Here's how the part is built. I have some questions about the finished solid (model axes, mm). Face numbers are marked on the shaded views. A direction names the side the tool comes from. Round coordinates to 2 decimals unless told otherwise and drop trailing zeros. Order: outer loops, then holes, each group sorted by start corner. A loop starts at its lowest first (then second) coordinate and runs counter-clockwise, first axis right, second up. Notation, with made-up numbers: (-5, -5.5) -> (39, -5.5) arc R18 cw to (39, 2.5) -> close; hole circle Ø6 at (-22.75, 39). An arc over 180 degrees is marked (long way). One line per item, written item: value.
```python
from build123d import *

# Parameters (mm, degrees)
SKETCH1_W           = 248.68
SKETCH1_H           = 10
BOSS_EXTRUDE1_DEPTH = 80
SKETCH3_W           = 10
SKETCH3_H           = 248.68
BOSS_EXTRUDE2_DEPTH = 40
SKETCH5_W           = 10
SKETCH5_H           = 248.68
BOSS_EXTRUDE3_DEPTH = 50
FILLET1_R           = 11
FILLET2_R           = 11
SKETCH6_W           = 227.416539417
SKETCH6_H           = 3
CUT_EXTRUDE2_DEPTH  = 70


with BuildPart() as part:
    # Sketch1 → Boss-Extrude1 (new body)
    with BuildSketch(Plane(origin=(0, 0, 0), x_dir=(0, 0, -1), z_dir=(1, 0, 0))):
        with Locations((117.31979798, -0.946969697)):
            Rectangle(SKETCH1_W, SKETCH1_H)
    extrude(amount=BOSS_EXTRUDE1_DEPTH)

    # Sketch3 → Boss-Extrude2 (add)
    with BuildSketch(Plane(origin=(0, 4.053030303, 0), x_dir=(1, 0, 0), z_dir=(0, 1, 0))):
        with Locations((5, 117.31979798)):
            Rectangle(SKETCH3_W, SKETCH3_H)
    extrude(amount=BOSS_EXTRUDE2_DEPTH)

    # Sketch5 → Boss-Extrude3 (add)
    with BuildSketch(Plane.XZ.offset(5.946969697)):
        with Locations((5, -117.31979798)):
            Rectangle(SKETCH5_W, SKETCH5_H)
    extrude(amount=BOSS_EXTRUDE3_DEPTH)

    # Fillet1
    # the kernel refuses this fillet: 11 mm, written as the material it takes off along each edge
    with BuildSketch(Plane(origin=(10, 44.053030303, -269.045925855), x_dir=(-1, 0, 0), z_dir=(0, 0, 1))) as fillet1_piece_1:
        with BuildLine():
            CenterArc((11, 10.95445115), FILLET1_R, 180, 84.78409143)
            Line((0, 10.95445115), (-0.22, 10.95445115))
            Line((-0.22, 10.95445115), (-0.22, 0))
            Line((-0.22, 0), (0, -0.22))
            ThreePointArc((0, -0.22), (5, -0.22), (9.98, -0.219089023))
            Line((9.98, -0.219089023), (10, 0))
        make_face()
    extrude(amount=303.452255751, mode=Mode.SUBTRACT)

    # Fillet2
    # the kernel refuses this fillet: 11 mm, written as the material it takes off along each edge
    with BuildSketch(Plane(origin=(10, -55.946969697, 34.406329895), x_dir=(-1, 0, 0), z_dir=(0, 0, -1))) as fillet2_piece_1:
        with BuildLine():
            CenterArc((11, 10.95445115), FILLET2_R, 180, 84.78409143)
            Line((0, 10.95445115), (-0.22, 10.95445115))
            Line((-0.22, 10.95445115), (-0.22, 0))
            Line((-0.22, 0), (0, -0.22))
            ThreePointArc((0, -0.22), (5, -0.22), (9.98, -0.219089023))
            Line((9.98, -0.219089023), (10, 0))
        make_face()
    extrude(amount=303.452255751, mode=Mode.SUBTRACT)

    # Sketch6 → Cut-Extrude2 (cut)
    with BuildSketch(Plane(origin=(80, 0, 0), x_dir=(0, 0, -1), z_dir=(1, 0, 0))):
        with Locations((117.951528272, -0.946969697)):
            Rectangle(SKETCH6_W, SKETCH6_H)
    extrude(amount=-CUT_EXTRUDE2_DEPTH, mode=Mode.SUBTRACT)


solid = part.part
```
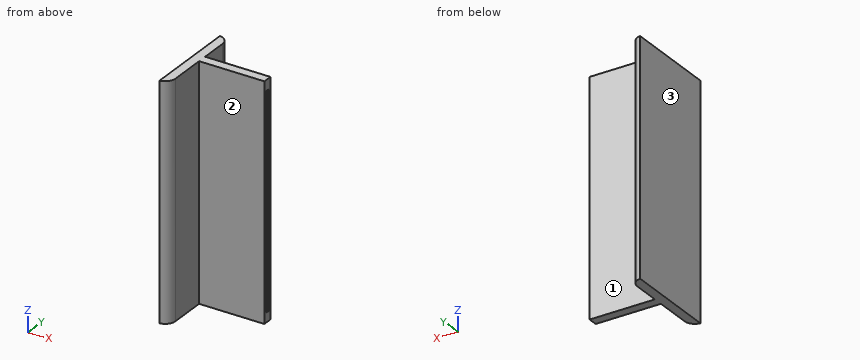
Q1. I want a section at B-B on z = -209. Write out the boundary of the cut face in (x, y).
Answers:
outline: (0, -55.95) arc R11 ccw to (10, -44.99) -> (10, -5.95) -> (80, -5.95) -> (80, -2.45) -> (10, -2.45) -> (10, 0.55) -> (80, 0.55) -> (80, 4.05) -> (10, 4.05) -> (10, 33.1) arc R11 ccw to (0, 44.05) -> close
Q2. I need wall thicknesses on line 1 along Y through (x, z) = (14.5, -163.5); line 2 along X through (y, z) = (23, -104); line 3 along Y through (x, z) = (5.5, -142.5). Which ranges of each line are inside material? Lowest first, please.
Answers:
line 1: -5.95 to -2.45, 0.55 to 4.05
line 2: 0 to 10
line 3: -53.87 to 41.97
Q3. Which directions (+Z, -Z, +X, -X, +Y, -Y) give clear straight access to the entire face, cutting with the end or side of a thin tool? Please do the marked faces 1, 2 and 3.
Answers:
face 1: +Z, -Z, +X, +Y
face 2: +Z, -Z, +X, -Y
face 3: +Z, -Z, -X, +Y, -Y
Q4. I want a section at C-C on y = -23. Write out the boundary of the cut face in (x, z), then the cut area to 3 significant figures.
Answers:
outline: (0, -241.66) -> (10, -241.66) -> (10, 7.02) -> (0, 7.02) -> close
area: 2,490 mm2
Q5. For P1, Ø14.5, axis at y = 22.5, z = -85.5, coming from the +X side; P2, Ø5, axis at x = 36, z = -42.5, coming from the -Y side; P3, Ø6, axis at x = 42, z = -140.5, coming from the +Y side; P4, Ø1.5, axis at y = -19, z = -158.5, coming from the -X side, each with a flat end and sliding along its axis, tell me the tip position at first contact or that it passes through.
Answers:
P1: x = 10
P2: y = -5.95
P3: y = 4.05
P4: x = 0
Q6. I want a section at A-A on x = 40.5. Write out the boundary of the cut face in (y, z), then the cut area to 3 significant figures.
Answers:
outline: (-5.95, -241.66) -> (4.05, -241.66) -> (4.05, 7.02) -> (-5.95, 7.02) -> close; hole (-2.45, -231.66) -> (0.55, -231.66) -> (0.55, -4.24) -> (-2.45, -4.24) -> close
area: 1,800 mm2
